from build123d import *

# Parameters (mm, degrees)
SKETCH1_R           = 2.5
BOSS_EXTRUDE1_DEPTH = 9
SKETCH2_R           = 3
BOSS_EXTRUDE3_DEPTH = 1
FILLET3_R           = 2.25
SKETCH4_R           = 0.224891602
BOSS_EXTRUDE4_DEPTH = 3


with BuildPart() as part:
    # Sketch1 → Boss-Extrude1 (new body)
    with BuildSketch(Plane(origin=(0, 0, 0), x_dir=(1, 0, 0), z_dir=(0, 1, 0))):
        with Locations(Location((0, 0, 0), (0, 0, 270))):  # turned: the seam where the file's is
            Circle(SKETCH1_R)
    extrude(amount=BOSS_EXTRUDE1_DEPTH)

    # Sketch2 → Boss-Extrude3 (add)
    with BuildSketch(Plane(origin=(0, 9, 0), x_dir=(1, 0, 0), z_dir=(0, 1, 0))):
        with Locations(Location((0, 0, 0), (0, 0, 270))):  # turned: the seam where the file's is
            Circle(SKETCH2_R)
    extrude(amount=-BOSS_EXTRUDE3_DEPTH)

    # Fillet3
    fillet3_edges = [part.edges().sort_by_distance(p)[0] for p in [
        (0, 0, -2.5),
    ]]
    fillet(fillet3_edges, radius=FILLET3_R)

    # Sketch4 → Boss-Extrude4 (add)
    with BuildSketch(Plane(origin=(0, 9, 0), x_dir=(1, 0, 0), z_dir=(0, 1, 0))):
        with Locations(Location((-2.366051797, 0, 0), (0, 0, 270))):  # turned: the seam where the file's is
            Circle(SKETCH4_R)
        with Locations(Location((-0.756710259, 0, 0), (0, 0, 270))):  # turned: the seam where the file's is
            Circle(SKETCH4_R)
        with Locations(Location((0.959210188, 0, 0), (0, 0, 270))):  # turned: the seam where the file's is
            Circle(SKETCH4_R)
        with Locations(Location((2.472630707, 0, 0), (0, 0, 270))):  # turned: the seam where the file's is
            Circle(SKETCH4_R)
    extrude(amount=BOSS_EXTRUDE4_DEPTH)


solid = part.part
Can you work these out from the model? Positions are in its coordinate system, mm. A direction names the side the tool comes from. Coordinates: 2 decimals unless noted, no trailing zeros. Write each loop counter-clockwise with the first axis right and the second up, starting at its lowest first coordinate (ties: lowest second). Pieces come first, ordered by that corner, then holes. Notation, with made-up numbers: (86, 34) - (98, 34) arc R5 ccw to (98, 41) - close; hole circle Ø5 at (86.25, 15.5). An arc over 180 degrees is marked (long way). Return JSON: item names as keys, results as strings. Group by question number.
Item 1: If we section it at A-A (y = 5.25): Write out the boundary of the cut face in (x, z).
Item 2: I'm going to push flat-ended pins straight in: pin 1 Ø2 at (x, y) = (2, 2.5) entering from -Z; pin 2 Ø3 at (x, y) = (-0.5, 2) entering from -Z; pin 3 Ø2 at (x, z) = (-0.5, 2) entering from -Y. Where does each tip first touch, or does it pass through?
Item 3: Which directions (+Z, -Z, +X, -X, +Y, -Y) give clear straight access to the entire face, cutting with the end or side of a thin tool? Please do faces 1 (the face through (2, 8, -2)), 2 (the face through (0.9, 8.51, 2.86)).
Item 4: Please list where these lines run through material, in increasing order: probe 1 along Y at (x, z) = (-2.35, 1); probe 2 along Z at (x, y) = (0, 7.5); probe 3 along Y at (x, z) = (-1.8, 0.2).
Return value:
{
 "1": {"outline": "circle Ø5 at (0, 0)"},
 "2": {"pin 1": "stops at z = -2.29", "pin 2": "stops at z = -2.5", "pin 3": "stops at y = 0.15"},
 "3": {"face 1": "-Y", "face 2": "+Y, -Y"},
 "4": {"probe 1": "y = 8 to 9", "probe 2": "z = -2.5 to 2.5", "probe 3": "y = 0.63 to 9"}
}
